Input: part model. Units: mm. Frame: model coordinates. A direction names the side the tool comes from. Round coordinates to 2 decimals unless told otherwise and drop trailing zeros. Write each loop counter-clockwise with the first axis right and the second up, starting at its lowest first coordinate (ties: lowest second). Pieces come first, ordered by that corner, then holes. Notation, with made-up numbers: (-28, -29.5) -> (-15, -29.5) arc R31 cw to (-15, 0.5) -> close; hole circle Ø9 at (9, 28.25). An arc over 180 degrees is marked (long way). Write item = value, one per line.
Autodesk Inventor part; units mm, degrees
ref_plane "YZ Plane" through (0, 0, 0) normal (1, 0, 0) x (0, 1, 0)
ref_plane "XZ Plane" through (0, 0, 0) normal (0, 1, 0) x (-1, 0, 0)
ref_plane "XY Plane" through (0, 0, 0) normal (0, 0, 1) x (1, 0, 0)
sketch "Sketch4" plane through (0, 0, 0) normal (1, 0, 0) x (0, 1, 0)
  line L0 (0, 0) -> (5.5, 0)
  line L1 (5.5, 0) -> (5.5, 6.6)
  line L2 (5.5, 6.6) -> (0, 6.6)
  line L3 (0, 6.6) -> (0, 0)
  line L4 (5.5, 5.8) -> (10.5, 5.8)
  line L5 (10.5, 5.8) -> (10.5, 0.8)
  line L6 (10.5, 0.8) -> (5.5, 0.8)
  line L7 (5.5, 0.8) -> (5.5, 5.8)
  line L8 (0, 3.3) -> (20.5, 3.3)
  line L9 (10.5, 5.3) -> (20.5, 5.3)
  line L10 (20.5, 5.3) -> (20.5, 1.3)
  line L11 (20.5, 1.3) -> (10.5, 1.3)
  line L12 (10.5, 1.3) -> (10.5, 5.3)
  dimension "d0" = 6.6
  dimension "d1" = 5.5
  dimension "d2" = 5
  dimension "d3" = 4
  dimension "d4" = 15
  dimension "d5" = 10
extrude "Extrusion1" add sketch "Sketch4" along normal blind 2
fillet "Fillet1" radius 0.5 8 edges at (1, 10.5, 5.3) (1, 20.5, 5.3) (1, 10.5, 5.8) (1, 20.5, 1.3) (1, 10.5, 1.3) (1, 10.5, 0.8) (1, 5.5, 0) (1, 5.5, 6.6)
fillet "Fillet2" radius 0.2 18 edges at (2, 10.3837, 5.7329) (2, 15.4995, 5.3) (2, 20.3536, 5.1536) (2, 20.5, 3.3) (2, 20.3536, 1.4464) (2, 15.4995, 1.3) (2, 10.3837, 0.8671) (2, 7.8168, 0.8) (2, 7.8168, 5.8) (0, 10.3837, 5.7329) (0, 15.4995, 5.3) (0, 20.3536, 5.1536) (0, 20.5, 3.3) (0, 20.3536, 1.4464) (0, 15.4995, 1.3) (0, 10.3837, 0.8671) (0, 7.8168, 0.8) (0, 7.8168, 5.8)
properties part number "Slider"
1) Access query for faces 1 (the face through (1, 2, 0)), 2 (the face through (1, 8, 0.8)), 3 (the face through (1, 15, 5.3)). Directions: +Z, -Z, +X, -X, +Y, -Y. A direction counts if a zero-diameter tool reaches every point of the face in a straight line with its end or side. Return the directions, or none.
Solutions:
face_1 = -Z, +X, -X, +Y, -Y
face_2 = -Z, +X, -X, +Y
face_3 = +Z, +X, -X, +Y
2) First-contact query: P1, Ø0.8, axis at x = 1, y = 16.5, coming from the -Z side. Flat tip, straight axial feed; report the tip coordinate or a pass-through.
Solutions:
P1 = 1.3
3) Cut plane B-B (y = 5.75). Return the cut outline in (x, z), and give its area (3 significant figures).
Solutions:
outline = (0, 1) arc R0.2 ccw to (0.2, 0.8) -> (1.8, 0.8) arc R0.2 ccw to (2, 1) -> (2, 5.6) arc R0.2 ccw to (1.8, 5.8) -> (0.2, 5.8) arc R0.2 ccw to (0, 5.6) -> close
area = 9.97 mm^2
4) Line query: L1, parallel to Z at x = 0.55, y = 18.25; L2, parallel to Z at x = 0.5, y = 9; L3, parallel to Y at x = 1.65, z = 0.5. Output: solid intervals per line, ascending. Write a range as from..to.
Solutions:
L1 = 1.3..5.3
L2 = 0.8..5.8
L3 = 0..5.5
5) Cut plane A-A (y = 13.75). Return the cut outline in (x, z).
Solutions:
outline = (0, 1.5) arc R0.2 ccw to (0.2, 1.3) -> (1.8, 1.3) arc R0.2 ccw to (2, 1.5) -> (2, 5.1) arc R0.2 ccw to (1.8, 5.3) -> (0.2, 5.3) arc R0.2 ccw to (0, 5.1) -> close
